Geometry check sheet. Reference: drawing and pictorial views, mm from the part's lowest x, y, z. Coordinates: 2 decimals unless noted, no trailing zeros. Write each loop counter-clockwise with the first axis right and the second up, starting at its lowest first coordinate (ties: lowest second). Pieces come first, ordered by that corner, then holes. Notation, with made-up numbers: (14, 81.5) -> (55, 81.5) arc R15 ccw to (55, 107.5) -> close; hole circle Ø8 at (-30.5, 7). An arc over 180 degrees is marked (long way). Use a Markdown table: item, result. Add a question column.
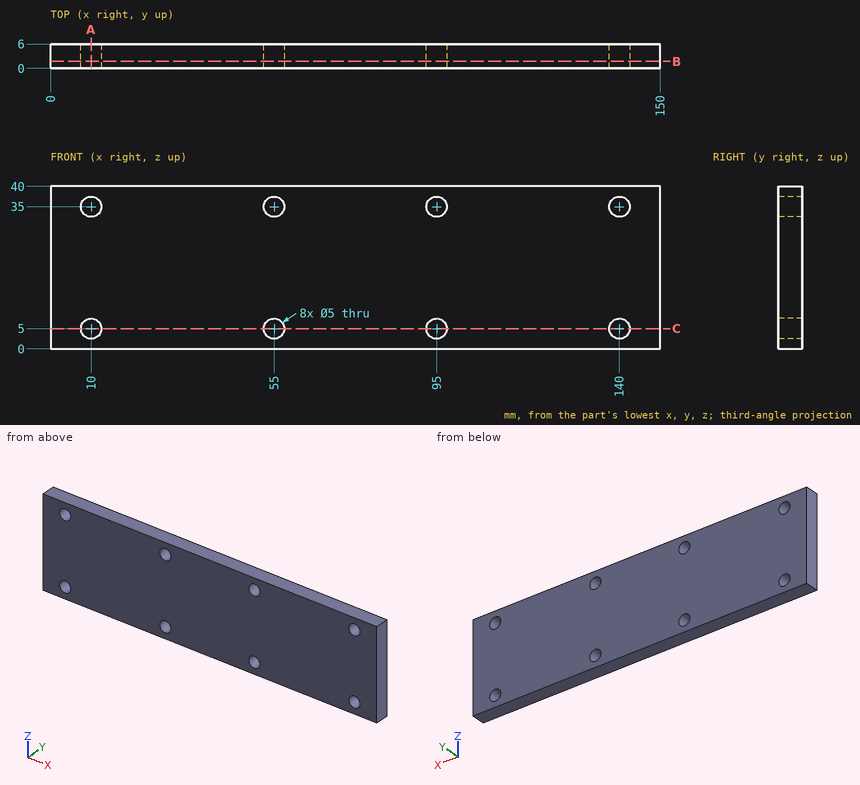
1) Gauge pin test, flat end, axial feed: pin 1 (4 mm diameter, centred on x = 10, z = 35, fed in from -Y). Record the tip position at first contact, or that the pin passes through.
2) Cross-section at B-B on y = 1.75. Give the number of separate pieces and of enclosed holes in the cut face, then the cut area to 3 significant figures.
3) Cross-section at A-A on x = 10. Record the boundary of the cut face in (y, z), then the cut area to 3 significant figures.
4) Thickness scan on L1, parallel to Z at x = 140, y = 5.2; L2, parallel to X at y = 3.9, z = 3; L3, parallel to X at y = 4.8, z = 6. Record the ranges inside material, lowest first.
5) Cross-section at C-C on z = 5. Record the boundary of the cut face in (x, y).
Returned:
| question | item | result |
|---|---|---|
| 1 | pin 1 | passes through |
| 2 | separate pieces | 1 |
| 2 | enclosed holes | 8 |
| 2 | area | 5,840 mm² |
| 3 | outline | (0, 0) -> (6, 0) -> (6, 2.5) -> (0, 2.5) -> close; (0, 7.5) -> (6, 7.5) -> (6, 32.5) -> (0, 32.5) -> close; (0, 37.5) -> (6, 37.5) -> (6, 40) -> (0, 40) -> close |
| 3 | area | 180 mm² |
| 4 | L1 | z = 0 to 2.5, 7.5 to 32.5, 37.5 to 40 |
| 4 | L2 | x = 0 to 8.5, 11.5 to 53.5, 56.5 to 93.5, 96.5 to 138.5, 141.5 to 150 |
| 4 | L3 | x = 0 to 7.71, 12.29 to 52.71, 57.29 to 92.71, 97.29 to 137.71, 142.29 to 150 |
| 5 | outline | (0, 0) -> (7.5, 0) -> (7.5, 6) -> (0, 6) -> close; (12.5, 0) -> (52.5, 0) -> (52.5, 6) -> (12.5, 6) -> close; (57.5, 0) -> (92.5, 0) -> (92.5, 6) -> (57.5, 6) -> close; (97.5, 0) -> (137.5, 0) -> (137.5, 6) -> (97.5, 6) -> close; (142.5, 0) -> (150, 0) -> (150, 6) -> (142.5, 6) -> close |
